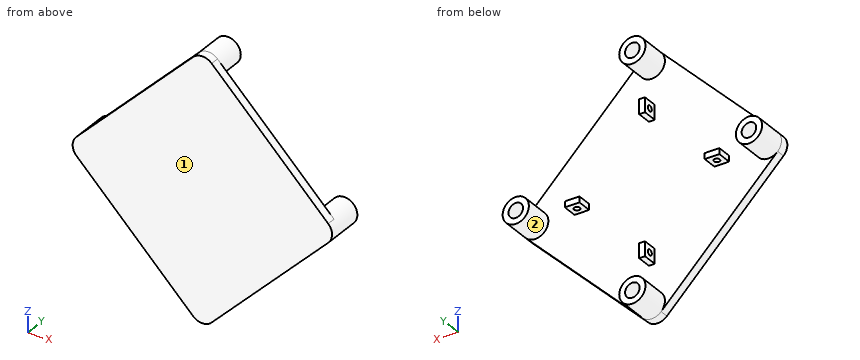
```python
from build123d import *

# Parameters (mm, degrees)
SKETCH1_W           = 100
SKETCH1_H           = 100
BOSS_EXTRUDE1_DEPTH = 3
SKETCH2_R           = 4.5
SKETCH2_R_2         = 2.5
BOSS_EXTRUDE2_DEPTH = 10
SKETCH3_W           = 4.999999906
SKETCH3_H           = 2
SKETCH3_W_2         = 2
SKETCH3_H_2         = 4.999999906
BOSS_EXTRUDE3_DEPTH = 5
CUT_EXTRUDE1_REACH  = 53
SKETCH4_R           = 1
CUT_EXTRUDE2_REACH  = 53
SKETCH5_R           = 1
CUT_EXTRUDE3_REACH  = 53
SKETCH7_R           = 1
CUT_EXTRUDE4_REACH  = 53
SKETCH8_R           = 1
SKETCH9_OUTSIDE_W   = 130.404
SKETCH9_OUTSIDE_H   = 130.404
CUT_EXTRUDE5_DEPTH  = 127


with BuildPart() as part:
    # Sketch1 → Boss-Extrude1 (new body)
    with BuildSketch(Plane(origin=(0, 0, 0), x_dir=(1, 0, 0), z_dir=(0, 1, 0))):
        Rectangle(SKETCH1_W, SKETCH1_H)
    extrude(amount=BOSS_EXTRUDE1_DEPTH)

    # Sketch2 → Boss-Extrude2 (add)
    with BuildSketch(Plane(origin=(0, 3, 0), x_dir=(1, 0, 0), z_dir=(0, 1, 0))):
        with Locations((0, 40)):
            Circle(SKETCH2_R)
        with Locations((0, 40)):
            Circle(SKETCH2_R_2, mode=Mode.SUBTRACT)
        with Locations((40, 0)):
            Circle(SKETCH2_R)
        with Locations((40, 0)):
            Circle(SKETCH2_R_2, mode=Mode.SUBTRACT)
        with Locations((0, -40)):
            Circle(SKETCH2_R)
        with Locations((0, -40)):
            Circle(SKETCH2_R_2, mode=Mode.SUBTRACT)
        with Locations((-40, 0)):
            Circle(SKETCH2_R)
        with Locations((-40, 0)):
            Circle(SKETCH2_R_2, mode=Mode.SUBTRACT)
    extrude(amount=BOSS_EXTRUDE2_DEPTH)

    # Sketch3 → Boss-Extrude3 (add)
    with BuildSketch(Plane(origin=(0, 3, 0), x_dir=(1, 0, 0), z_dir=(0, 1, 0))):
        with Locations((24.000000006, 0)):
            Rectangle(SKETCH3_W, SKETCH3_H)
        with Locations((0, 24.000000006)):
            Rectangle(SKETCH3_W_2, SKETCH3_H_2)
        with Locations((0, -24.000000006)):
            Rectangle(SKETCH3_W_2, SKETCH3_H_2)
        with Locations((-24.000000006, 0)):
            Rectangle(SKETCH3_W, SKETCH3_H)
    extrude(amount=BOSS_EXTRUDE3_DEPTH)

    # Sketch4 → Cut-Extrude1 (cut, up to next)
    with BuildSketch(Plane(origin=(1, 0, 0), x_dir=(0, 0, -1), z_dir=(1, 0, 0)), mode=Mode.PRIVATE) as cut_extrude1_sk1:
        with Locations((24.000000006, 5.5)):
            Circle(SKETCH4_R)
    cut_extrude1_tool1 = extrude(cut_extrude1_sk1.sketch, amount=-CUT_EXTRUDE1_REACH, mode=Mode.PRIVATE) & part.part
    add(cut_extrude1_tool1.solids().sort_by_distance((1, 5.5, -24))[0], mode=Mode.SUBTRACT)

    # Sketch5 → Cut-Extrude2 (cut, up to next)
    with BuildSketch(Plane(origin=(0, 0, -1), x_dir=(-1, 0, 0), z_dir=(0, 0, -1)), mode=Mode.PRIVATE) as cut_extrude2_sk1:
        with Locations((24.000000006, 5.5)):
            Circle(SKETCH5_R)
    cut_extrude2_tool1 = extrude(cut_extrude2_sk1.sketch, amount=-CUT_EXTRUDE2_REACH, mode=Mode.PRIVATE) & part.part
    add(cut_extrude2_tool1.solids().sort_by_distance((-24, 5.5, -1))[0], mode=Mode.SUBTRACT)

    # Sketch7 → Cut-Extrude3 (cut, up to next)
    with BuildSketch(Plane.ZY.offset(1), mode=Mode.PRIVATE) as cut_extrude3_sk1:
        with Locations((24.000000006, 5.5)):
            Circle(SKETCH7_R)
    cut_extrude3_tool1 = extrude(cut_extrude3_sk1.sketch, amount=-CUT_EXTRUDE3_REACH, mode=Mode.PRIVATE) & part.part
    add(cut_extrude3_tool1.solids().sort_by_distance((-1, 5.5, 24))[0], mode=Mode.SUBTRACT)

    # Sketch8 → Cut-Extrude4 (cut, up to next)
    with BuildSketch(Plane.XY.offset(1), mode=Mode.PRIVATE) as cut_extrude4_sk1:
        with Locations((24.000000006, 5.5)):
            Circle(SKETCH8_R)
    cut_extrude4_tool1 = extrude(cut_extrude4_sk1.sketch, amount=-CUT_EXTRUDE4_REACH, mode=Mode.PRIVATE) & part.part
    add(cut_extrude4_tool1.solids().sort_by_distance((24, 5.5, 1))[0], mode=Mode.SUBTRACT)

    # Sketch9 outside → Cut-Extrude5 (cut)
    with BuildSketch(Plane(origin=(0, 3, 0), x_dir=(1, 0, 0), z_dir=(0, 1, 0))):
        Rectangle(SKETCH9_OUTSIDE_W, SKETCH9_OUTSIDE_H)
        with BuildLine():
            Line((3.181980515, 43.181980515), (43.181980515, 3.181980515))
            ThreePointArc((43.181980515, 3.181980515), (44.5, 0), (43.181980515, -3.181980515))
            Line((43.181980515, -3.181980515), (3.181980515, -43.181980515))
            ThreePointArc((3.181980515, -43.181980515), (0, -44.5), (-3.181980515, -43.181980515))
            Line((-3.181980515, -43.181980515), (-43.181980515, -3.181980515))
            ThreePointArc((-43.181980515, -3.181980515), (-44.5, 0), (-43.181980515, 3.181980515))
            Line((-43.181980515, 3.181980515), (-3.181980515, 43.181980515))
            ThreePointArc((-3.181980515, 43.181980515), (0, 44.5), (3.181980515, 43.181980515))
        make_face(mode=Mode.SUBTRACT)
    extrude(amount=-CUT_EXTRUDE5_DEPTH, mode=Mode.SUBTRACT)


solid = part.part
```
The model under review builds one solid part; all positions refer to its coordinate system, in mm. Face numbers are marked on the shaded views. Round coordinates to 2 decimals unless told otherwise and drop trailing zeros. Order: outer loops, then holes, each group sorted by start corner. A loop starts at its lowest first (then second) coordinate and runs counter-clockwise, first axis right, second up. Notation, with made-up numbers: (-17.75, -25) -> (4.25, -25) arc R21 ccw to (4.25, -19) -> close; hole circle Ø8 at (-24.5, 51). An arc over 180 degrees is marked (long way). One line per item, written item: value. Start each with the question number.
Q1. Take a section at D-D (z = 9.5). Write out the cut boundary in (x, y).
Q2. Take a section at A-A (y = 11.5). Write out the cut boundary in (x, z), and give its area (3 significant figures).
Q3. Take a section at B-B (z = 40). Write out the cut boundary in (x, y), and give its area (3 significant figures).
Q4. Take a section at C-C (x = 40). Write out the cut boundary in (y, z), and give its area (3 significant figures).
Q5. Mouldability with a two-part tool opening along X and no side actions: class the marked faces 1 and 2 as released by +X, released by -X, zero draft, split by the parting line, or undercut.
Q6. Clearance check with flat-ended pins moving along their axes: pin 1 Ø5 at (x, y) = (3, 4.5) entering from -Z; pin 2 Ø2.5 at (y, z) = (5.5, -24) entering from -X; pin 3 Ø1.5 at (x, y) = (-3, 7.5) entering from +Z. State where each tip first meets the part, or that it passes through.
Q7. Wall thickness on line 1 (Z direction, x = 40, y = 6); line 2 (Z direction, x = -1, y = 12); line 3 (Y direction, x = -0.2, z = 24): over which ranges is each line inside the solid? List them lowest first.
Reported:
1. outline: (-36.86, 0) -> (36.86, 0) -> (36.86, 3) -> (-36.86, 3) -> close
2. outline: circle Ø9 at (-40, 0); circle Ø9 at (0, -40); circle Ø9 at (0, 40); circle Ø9 at (40, 0); hole circle Ø5 at (-40, 0); hole circle Ø5 at (0, -40); hole circle Ø5 at (0, 40); hole circle Ø5 at (40, 0)
2. area: 176 mm2
3. outline: (-6.36, 0) -> (6.36, 0) -> (6.36, 3) -> (4.5, 3) -> (4.5, 13) -> (2.5, 13) -> (2.5, 3) -> (-2.5, 3) -> (-2.5, 13) -> (-4.5, 13) -> (-4.5, 3) -> (-6.36, 3) -> close
3. area: 78.2 mm2
4. outline: (0, -6.36) -> (3, -6.36) -> (3, -4.5) -> (13, -4.5) -> (13, -2.5) -> (3, -2.5) -> (3, 2.5) -> (13, 2.5) -> (13, 4.5) -> (3, 4.5) -> (3, 6.36) -> (0, 6.36) -> close
4. area: 78.2 mm2
5. face 1: zero draft
5. face 2: undercut
6. pin 1: stops at z = -44.47
6. pin 2: stops at x = -1
6. pin 3: stops at z = 43.9
7. line 1: z = -4.5 to -2.5, 2.5 to 4.5
7. line 2: z = -44.39 to -42.29, -37.71 to -35.61, 35.61 to 37.71, 42.29 to 44.39
7. line 3: y = 0 to 4.5, 6.5 to 8
